Source: CAD feature listing. Evaluate the final solid. Frame: model axes, mm. A direction names the side the tool comes from. Round coordinates to 2 decimals unless told otherwise and drop trailing zeros. Loops run counter-clockwise (first coordinate to the right, second up) from the corner with the lowest first, then second, coordinate; pieces in that order, holes last. Notation, with made-up numbers: (50.5, -24) - (64.5, -24) arc R20 ccw to (64.5, -12) - close; hole circle Ø11 at (-30.75, 25). An arc over 180 degrees is marked (long way). One line per question, with ' | ' between items. Start each with the question number.
1. Cut plane A-A (x = 14.5). Return loops of the section in (y, z), then the cut area to 3 significant figures.
2. Ray query, line 1 (Y direction, x = 159, z = 15.5); line 2 (Y direction, x = 26, z = 3.75); line 3 (X direction, y = 10, z = 16.5). Return the intervals inside material, ascending.
3. Cut plane B-B (y = -53.5). Return loops of the section in (x, z).
4. Mould query, pull axis X, two halves, no side actions, for faces 1 (the flat face through (118, -27, 0)), 2 (the cylindrical face through (-16.8, -50.7, 12.3)), 3 (the cylindrical face through (77.313, -104.87, 12.325)). Classes: pulls with the +X half, pulls with the -X half, needs draft (parallel to the pull), parting line crosses it, or undercut.
5. Cut plane C-C (x = 106). Return loops of the section in (y, z).
6. Access query for faces 4 (the flat face through (182, 32.279, 12)), 5 (the flat face through (21, 52.279, 12)), 6 (the flat face through (70.321, 12, 12)). Directions: +Z, -Z, +X, -X, +Y, -Y. A direction counts if a zero-diameter tool reaches every point of the face in a straight line with its end or side. Return the directions, or none.
7. Pin query (flat end, axial travel): pin 1 (7.5 mm diameter, centred on x = 210.5, z = 7, fed in from +Y); pin 2 (12.5 mm diameter, centred on x = 163.5, z = 12.5, fed in from -Y); pin 3 (6 mm diameter, centred on y = -64, z = 18.5, fed in from +X). Return the tip coordinate at first contact, or that it passes through.
8. Cut plane D-D (y = -82.5). Return loops of the section in (x, z), then the cut area to 3 significant figures.
```python
from build123d import *

# Parameters (mm, degrees)
F1_DEPTH = 25


with BuildPart() as f1:
    # F0 (on Top) → F1 (new body)
    with BuildSketch(Plane.XY):
        with BuildLine():
            ThreePointArc((-29.679486, 52.278812), (-36.750554, 49.34988), (-39.679486, 42.278812))
            Line((-39.679486, 42.278812), (-39.679486, -97.721188))
            ThreePointArc((-39.679486, -97.721188), (-36.750554, -104.792256), (-29.679486, -107.721188))
            Line((-29.679486, -107.721188), (70.320514, -107.721188))
            ThreePointArc((70.320514, -107.721188), (77.391582, -104.792256), (80.320514, -97.721188))
            Line((80.320514, -97.721188), (80.320514, -77.721188))
            ThreePointArc((80.320514, -77.721188), (83.249446, -70.65012), (90.320514, -67.721188))
            Line((90.320514, -67.721188), (270.320514, -67.721188))
            ThreePointArc((270.320514, -67.721188), (277.391582, -64.792256), (280.320514, -57.721188))
            Line((280.320514, -57.721188), (280.320514, 22.278812))
            ThreePointArc((280.320514, 22.278812), (277.391582, 29.34988), (270.320514, 32.278812))
            Line((270.320514, 32.278812), (90.320514, 32.278812))
            ThreePointArc((90.320514, 32.278812), (83.249446, 35.207744), (80.320514, 42.278812))
            ThreePointArc((80.320514, 42.278812), (77.391582, 49.34988), (70.320514, 52.278812))
            Line((70.320514, 52.278812), (-29.679486, 52.278812))
        make_face()
        with BuildLine():
            ThreePointArc((-19.679486, -57.721188), (-16.750554, -50.65012), (-9.679486, -47.721188))
            Line((-9.679486, -47.721188), (60.320514, -47.721188))
            ThreePointArc((60.320514, -47.721188), (67.391582, -50.65012), (70.320514, -57.721188))
            Line((70.320514, -57.721188), (70.320514, -77.721188))
            ThreePointArc((70.320514, -77.721188), (67.391582, -84.792256), (60.320514, -87.721188))
            Line((60.320514, -87.721188), (-9.679486, -87.721188))
            ThreePointArc((-9.679486, -87.721188), (-16.750554, -84.792256), (-19.679486, -77.721188))
            Line((-19.679486, -77.721188), (-19.679486, -57.721188))
        make_face(mode=Mode.SUBTRACT)
        with BuildLine():
            Line((259.320514, -58.89954), (85.204735, -58.89954))
            ThreePointArc((85.204735, -58.89954), (80.204735, -53.89954), (85.204735, -48.89954))
            Line((85.204735, -48.89954), (259.320514, -48.89954))
            ThreePointArc((259.320514, -48.89954), (264.320514, -53.89954), (259.320514, -58.89954))
        make_face(mode=Mode.SUBTRACT)
        with BuildLine():
            ThreePointArc((-19.679486, 22.278812), (-16.750554, 29.34988), (-9.679486, 32.278812))
            Line((-9.679486, 32.278812), (60.320514, 32.278812))
            ThreePointArc((60.320514, 32.278812), (67.391582, 29.34988), (70.320514, 22.278812))
            Line((70.320514, 22.278812), (70.320514, 2.278812))
            ThreePointArc((70.320514, 2.278812), (67.391582, -4.792256), (60.320514, -7.721188))
            Line((60.320514, -7.721188), (-9.679486, -7.721188))
            ThreePointArc((-9.679486, -7.721188), (-16.750554, -4.792256), (-19.679486, 2.278812))
            Line((-19.679486, 2.278812), (-19.679486, 22.278812))
        make_face(mode=Mode.SUBTRACT)
        with BuildLine():
            Line((259.320514, -26.34807), (83.129056, -26.34807))
            ThreePointArc((83.129056, -26.34807), (78.129056, -21.34807), (83.129056, -16.34807))
            Line((83.129056, -16.34807), (259.320514, -16.34807))
            ThreePointArc((259.320514, -16.34807), (264.320514, -21.34807), (259.320514, -26.34807))
        make_face(mode=Mode.SUBTRACT)
        with BuildLine():
            Line((258.52415, 4.408746), (81.572294, 4.408746))
            ThreePointArc((81.572294, 4.408746), (76.572294, 9.408746), (81.572294, 14.408746))
            Line((81.572294, 14.408746), (258.52415, 14.408746))
            ThreePointArc((258.52415, 14.408746), (263.52415, 9.408746), (258.52415, 4.408746))
        make_face(mode=Mode.SUBTRACT)
    extrude(amount=F1_DEPTH)


solid = f1.part
```
Answers follow:
1) outline: (-107.72, 0) - (-87.72, 0) - (-87.72, 25) - (-107.72, 25) - close; (-47.72, 0) - (-7.72, 0) - (-7.72, 25) - (-47.72, 25) - close; (32.28, 0) - (52.28, 0) - (52.28, 25) - (32.28, 25) - close | area: 2,000 mm2
2) line 1: y = -67.72 to -58.9, -48.9 to -26.35, -16.35 to 4.41, 14.41 to 32.28 | line 2: y = -107.72 to -87.72, -47.72 to -7.72, 32.28 to 52.28 | line 3: x = -39.68 to -19.68, 70.32 to 76.61, 263.49 to 280.32
3) outline: (-39.68, 0) - (-18.74, 0) - (-18.74, 25) - (-39.68, 25) - close; (69.39, 0) - (80.22, 0) - (80.22, 25) - (69.39, 25) - close; (264.3, 0) - (280.32, 0) - (280.32, 25) - (264.3, 25) - close
4) face 1: needs draft | face 2: undercut | face 3: pulls with the +X half
5) outline: (-67.72, 0) - (-58.9, 0) - (-58.9, 25) - (-67.72, 25) - close; (-48.9, 0) - (-26.35, 0) - (-26.35, 25) - (-48.9, 25) - close; (-16.35, 0) - (4.41, 0) - (4.41, 25) - (-16.35, 25) - close; (14.41, 0) - (32.28, 0) - (32.28, 25) - (14.41, 25) - close
6) face 4: +Z, -Z, +X, +Y | face 5: +Z, -Z, +X, -X, +Y | face 6: +Z, -Z
7) pin 1: stops at y = 32.28 | pin 2: stops at y = -67.72 | pin 3: stops at x = 279.77
8) outline: (-39.68, 0) - (-18.46, 0) - (-18.46, 25) - (-39.68, 25) - close; (69.1, 0) - (80.32, 0) - (80.32, 25) - (69.1, 25) - close | area: 811 mm2
